Geometry: final body of the model. Coordinates: model frame, mm. A direction names the side the tool comes from. Coordinates: 2 decimals unless noted, no trailing zeros. Loops run counter-clockwise (first coordinate to the right, second up) from the corner with the lowest first, then second, coordinate; pieces in that order, holes last. Notation, with made-up numbers: M 48,85 L 57,85 A34 ccw 57,115 Z; hole C -1.75,-25.75 d4. An arc over 180 degrees is marked long. Write each question's results on one line, items separated by ' | '. Start each with the question number.
from build123d import *

# Parameters (mm, degrees)
ESBO_O2_R             = 6
CORTE_EXTRUS_O1_DEPTH = 10
ESBO_O3_R             = 5
CORTE_EXTRUS_O2_DEPTH = 4


with BuildPart() as part:
    # Esboço1 → Revolução1 (revolve)
    with BuildSketch(Plane.XY):
        Polygon((0, 0), (0, 16.5), (8.5, 16.5), (7.5, 0), align=None)
    revolve(axis=Axis((0, 0, 0), (0, 1, 0)))

    # Esboço2 → Corte-extrusão1 (cut)
    with BuildSketch(Plane(origin=(0, 16.5, 0), x_dir=(1, 0, 0), z_dir=(0, 1, 0))):
        Circle(ESBO_O2_R)
    extrude(amount=-CORTE_EXTRUS_O1_DEPTH, mode=Mode.SUBTRACT)

    # Esboço3 → Corte-extrusão2 (cut)
    with BuildSketch(Plane.XZ):
        Circle(ESBO_O3_R)
    extrude(amount=-CORTE_EXTRUS_O2_DEPTH, mode=Mode.SUBTRACT)


solid = part.part
Item 1: Section A-A, the plane x = 0. Return loops of the section in (y, z).
Item 2: Ray query, L1, parallel to Z at x = 0, y = 13.25; L2, parallel to Z at x = 0, y = 9.5; L3, parallel to X at y = 9, z = 0. Return the intervals inside material, ascending. Write a range as [from, to].
Item 3: Section D-D, the plane y = 13. Return loops of the section in (x, z), plus the area to 3 significant figures.
Item 4: Section C-C, the plane y = 5. Return loops of the section in (x, z), plus the area to 3 significant figures.
Item 5: Section B-B, the plane z = 0. Return loops of the section in (x, y).
Item 6: Set-up query: faces 4 (the cylindrical face through (-1.08, 1.97, -4.88)), 5 (the cylindrical face through (-6, 12, 0)), 6 (the flat face through (-2, 16.5, -6)). Return all of +Z, -Z, +X, -X, +Y, -Y with unobstructed straight access to the full face (end or side cutting, diameter ignored); none if empty.
Item 7: Contact query for flat-ended pins moving along their axis: P1, Ø3.5, axis at x = -0.5, z = -2.5, coming from the +Y side; P2, Ø2, axis at y = 9, z = -4, coming from the +X side; P3, Ø8, axis at y = 3, z = 0, coming from the +X side. Output: stop coordinate, or through.
Item 8: Pull-direction query (Z, two-part tool) for faces 1 (the flat face through (0, 6.5, 0)), 2 (the flat face through (2, 0, 5)), 3 (the conical face through (-6.343, 8.134, 4.864)); classes: released by +Z, released by -Z, zero draft, split by the parting line, or undercut.
Solutions:
1) outline: M 0,-7.5 L 16.5,-8.5 L 16.5,-6 L 6.5,-6 L 6.5,6 L 16.5,6 L 16.5,8.5 L 0,7.5 L 0,5 L 4,5 L 4,-5 L 0,-5 Z
2) L1: z = [-8.3, -6], [6, 8.3] | L2: z = [-8.08, -6], [6, 8.08] | L3: x = [-8.05, -6], [6, 8.05]
3) outline: C 0,0 d16.58; hole C 0,0 d12 | area: 103 mm²
4) outline: C 0,0 d15.61 | area: 191 mm²
5) outline: M -8.5,16.5 L -7.5,0 L -5,0 L -5,4 L 5,4 L 5,0 L 7.5,0 L 8.5,16.5 L 6,16.5 L 6,6.5 L -6,6.5 L -6,16.5 Z
6) face 4: -Y | face 5: +Y | face 6: +Z, -Z, +X, -X, +Y
7) P1: stops at y = 6.5 | P2: stops at x = 7.47 | P3: stops at x = 7.92
8) face 1: undercut | face 2: zero draft | face 3: split by the parting line
